```python
from build123d import *

# Parameters (mm, degrees)
MAIN_W                         = 46.736
MAIN_H                         = 1689.1
EXTRUDE_MAIN_DEPTH             = 44.45
MAIN_CUT_W                     = 32.258
MAIN_CUT_H                     = 34.29
CUT_MAIN_DEPTH                 = 1690.846346839
SKETCH1_W                      = 3.937
SKETCH1_H                      = 44.45
CUT_EXTRUDE1_DEPTH             = 1690.846346839
F_4_0_209_DIAMETER_HOLE2_D     = 5.3086
F_4_0_209_DIAMETER_HOLE2_DEPTH = 5.461
FILLET1_R                      = 2.54


with BuildPart() as part:
    # Main → Extrude-Main (new body)
    with BuildSketch(Plane(origin=(0, 0, 0), x_dir=(1, 0, 0), z_dir=(0, 1, 0))):
        Rectangle(MAIN_W, MAIN_H)
    extrude(amount=EXTRUDE_MAIN_DEPTH)

    # Main Cut → Cut-Main (cut, through all)
    with BuildSketch(Plane.XY.offset(844.55)):
        with Locations((-2.159, 22.225)):
            Rectangle(MAIN_CUT_W, MAIN_CUT_H)
    extrude(amount=-CUT_MAIN_DEPTH, mode=Mode.SUBTRACT)

    # Sketch1 → Cut-Extrude1 (cut, through all)
    with BuildSketch(Plane.XY.offset(844.55)):
        with Locations((21.3995, 22.225)):
            Rectangle(SKETCH1_W, SKETCH1_H)
    extrude(amount=-CUT_EXTRUDE1_DEPTH, mode=Mode.SUBTRACT)

    # #4 (0.209) Diameter Hole2
    with Locations(Plane.ZY.offset(-13.97)):
        with Locations((831.85, 22.225), (-831.85, 22.225), (-791.21, 22.225), (791.21, 22.225)):
            Hole(F_4_0_209_DIAMETER_HOLE2_D / 2, depth=F_4_0_209_DIAMETER_HOLE2_DEPTH)

    # Fillet1
    fillet1_edges = [part.edges().sort_by_distance(p)[0] for p in [
        (-23.368, 44.45, 0),
        (-18.288, 5.08, 0),
        (-18.288, 39.37, 0),
        (13.97, 39.37, 0),
        (13.97, 5.08, 0),
        (19.431, 0, 0),
        (19.431, 44.45, 0),
        (-23.368, 0, 0),
    ]]
    fillet(fillet1_edges, radius=FILLET1_R)


solid = part.part
```
Input: part model. Units: mm. Frame: model coordinates. A direction names the side the tool comes from. Give positions to 0.01 mm unless a question says otherwise; leave off trailing zeros. Order: outer loops, then holes, each group sorted by start corner. A loop starts at its lowest first (then second) coordinate and runs counter-clockwise, first axis right, second up. Notation, with made-up numbers: M 27,-30.75 L 41,-30.75 A28 cw 41,-9.75 Z; hole C 75.5,68 d5. An arc over 180 degrees is marked long. Return JSON: item names as keys, results as strings.
1) Access query for faces 1 (the face through (-18.288, 22, 12)), 2 (the face through (17, 22, 844.55)). Directions: +Z, -Z, +X, -X, +Y, -Y. A direction counts if a zero-diameter tool reaches every point of the face in a straight line with its end or side. Return the directions, or none.
Taken from the geometry:
{"face 1": "+Z, -Z", "face 2": "+Z, +X, -X, +Y, -Y"}
2) Contact query for a flat-ended pin moving along its axis: pin 1 (3 mm diameter, centred on y = 22.225, z = 791.21, fed in from +X). Output: stop coordinate, or through.
Taken from the geometry:
{"pin 1": "stops at x = -18.29"}
3) Mould query, pull axis Y, two halves, no side actions, for faces 3 (the face through (-2, 0, -12)), 4 (the face through (13.97, 22, 12)), 5 (the face through (-23.368, 22, 12)). Classes: released by +Y, released by -Y, zero draft, split by the parting line, or undercut.
Taken from the geometry:
{"face 3": "released by -Y", "face 4": "undercut", "face 5": "zero draft"}
4) Section query A-A on z = 647. Output: boundary loops of the cut face in (x, y).
Taken from the geometry:
{"outline": "M -23.37,2.54 A2.54 ccw -20.83,0 L 16.89,0 A2.54 ccw 19.43,2.54 L 19.43,41.91 A2.54 ccw 16.89,44.45 L -20.83,44.45 A2.54 ccw -23.37,41.91 Z; hole M -18.29,7.62 A2.54 ccw -15.75,5.08 L 11.43,5.08 A2.54 ccw 13.97,7.62 L 13.97,36.83 A2.54 ccw 11.43,39.37 L -15.75,39.37 A2.54 ccw -18.29,36.83 Z"}
5) Line query: L1, parallel to X at y = 36.5, z = 493; L2, parallel to Y at x = 5, z = -345; L3, parallel to Y at x = 17.65, z = -791.21. Output: solid intervals per line, ascending. Write a range as [from, to].
Taken from the geometry:
{"L1": "x = [-23.37, -18.29], [13.97, 19.43]", "L2": "y = [0, 5.08], [39.37, 44.45]", "L3": "y = [0.12, 19.57], [24.88, 44.33]"}
